Print and shaded views of the part. All mm, measured from the part's lowest x, y and z. A direction names the side the tool comes from. Round coordinates to 2 decimals unless told otherwise and drop trailing zeros. Loops run counter-clockwise (first coordinate to the right, second up) from the corner with the lowest first, then second, coordinate; pieces in that order, holes last. Notation, with made-up numbers: (1, 19) - (32, 19) arc R20 cw to (32, 40) - close; hole circle Ø8 at (14.5, 46.25). An arc over 180 degrees is marked (long way). Answer as a JSON object with one key per item and string values.
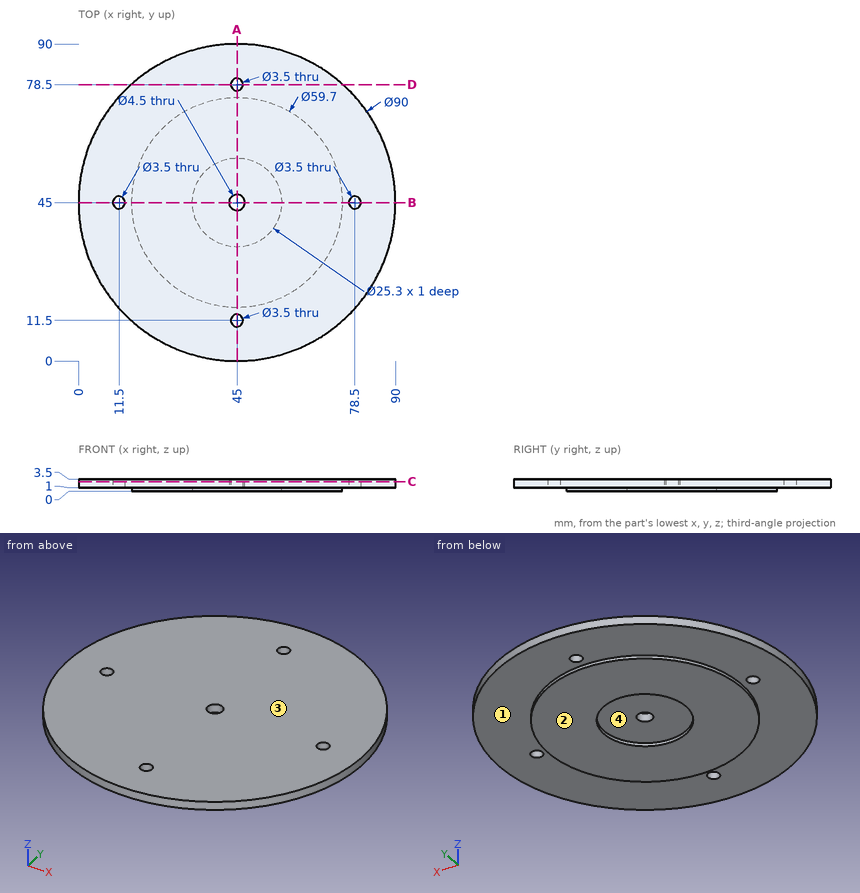
1) Tool access for the marked faces 1 and 2: list every direction of +Z, -Z, +X, -X, +Y, -Y with a clear straight run to the whole face (end or side of a thin tool).
Values follow:
{"face 1": "-Z", "face 2": "-Z, +X, -X, +Y, -Y"}
2) Slice it at A-A on x = 45. List the corners of the cut face in (y, z), then the cut area to 3 significant figures.
Values follow:
{"outline": "(0, 1) - (9.75, 1) - (9.75, 3.5) - (0, 3.5) - close; (13.25, 1) - (15.15, 1) - (15.15, 0) - (32.35, 0) - (32.35, 1) - (42.75, 1) - (42.75, 3.5) - (13.25, 3.5) - close; (47.25, 1) - (57.65, 1) - (57.65, 0) - (74.85, 0) - (74.85, 1) - (76.75, 1) - (76.75, 3.5) - (47.25, 3.5) - close; (80.25, 1) - (90, 1) - (90, 3.5) - (80.25, 3.5) - close", "area": "231 mm²"}
3) Two-plate mould, pull along Y, no slides. Class the marked faces 3 and 4: pulls with the +Y half, pulls with the -Y half, needs draft (parallel to the pull), parting line crosses it, or undercut.
Values follow:
{"face 3": "needs draft", "face 4": "undercut"}
4) Slice it at C-C on z = 2.75. List the corners of the cut face in (x, y), then the cut area to 3 significant figures.
Values follow:
{"outline": "circle Ø90 at (45, 45); hole circle Ø3.5 at (11.5, 45); hole circle Ø4.5 at (45, 45); hole circle Ø3.5 at (45, 11.5); hole circle Ø3.5 at (45, 78.5); hole circle Ø3.5 at (78.5, 45)", "area": "6,310 mm²"}
5) Probe probe 1 along Y at (x, z) = (45, 2.15); probe 2 along Z at (x, y) = (75.5, 40.5); probe 3 along Y at (x, z) = (45, 0.6). List the from-to ranges inside material, lowest first.
Values follow:
{"probe 1": "0 to 9.75, 13.25 to 42.75, 47.25 to 76.75, 80.25 to 90", "probe 2": "1 to 3.5", "probe 3": "15.15 to 32.35, 57.65 to 74.85"}
6) Drop flat-ended pins along their axis: P1, Ø1, axis at x = 19, y = 9, coming from the -Z side; P2, Ø3, axis at x = 11.5, y = 45, coming from the +Z side; P3, Ø1.5, axis at y = 35.5, z = 2.5, coming from the -X side; P4, Ø1, axis at y = 78, z = 2, coming from the -X side. Give the stop position or say it passes through.
Values follow:
{"P1": "z = 1", "P2": "through", "P3": "x = 0.86", "P4": "x = 13.88"}
7) Slice it at D-D on y = 78.5. List the corners of the cut face in (x, z), then the cut area to 3 significant figures.
Values follow:
{"outline": "(14.95, 1) - (43.25, 1) - (43.25, 3.5) - (14.95, 3.5) - close; (46.75, 1) - (75.05, 1) - (75.05, 3.5) - (46.75, 3.5) - close", "area": "141 mm²"}
